Could you check a few things on this model? Use its own coordinates, in mm. Face numbers are marked on the shaded views. Coordinates: 2 decimals unless noted, no trailing zeros. Write each loop counter-clockwise with the first axis right and the second up, starting at its lowest first coordinate (ties: lowest second). Pieces come first, ordered by that corner, then holes. Notation, with made-up numbers: M 17.5,-31 L 69.5,-31 A11 cw 69.5,-15 Z; hole C 75,25.25 d10. An arc over 180 degrees is marked long. Write item = value, one per line.
Autodesk Inventor part; units mm, degrees
ref_plane "YZ Plane" through (0, 0, 0) normal (1, 0, 0) x (0, 1, 0)
ref_plane "XZ Plane" through (0, 0, 0) normal (0, 1, 0) x (-1, 0, 0)
ref_plane "XY Plane" through (0, 0, 0) normal (0, 0, 1) x (1, 0, 0)
sketch "Sketch1" plane through (0, 0, 0) normal (0, 1, 0) x (-1, 0, 0)
  line L0 (15, 7.5) -> (-15, 7.5)
  line L1 (-15, 7.5) -> (-15, -7.5)
  line L2 (-15, -7.5) -> (15, -7.5)
  line L3 (15, -7.5) -> (15, 7.5)
  line L4 (15, 7.5) -> (-15, -7.5) construction
  line L5 (-15, 7.5) -> (15, -7.5) construction
  line L6 (0, 7.5) -> (0, -7.5)
  line L7 (15, 0) -> (0, 0)
  circle A0 centre (7.5, 0) radius 2.25
  circle A1 centre (-7.7235, 0) radius 2
  dimension "d0" = 30
  dimension "d1" = 15
  dimension "d2" = 4.5
  dimension "d11" = 4
extrude "Extrusion1" add sketch "Sketch1" along normal blind 5 contours L3 L7 A0 L6 L0 | L6 L2 L1 L0 | L3 L2 L6 L7 A0
fillet "Fillet1" radius 3 4 edges at (-15, 2.5, 7.5) (-15, 2.5, -7.5) (15, 2.5, 7.5) (15, 2.5, -7.5)
properties part number "angulo"
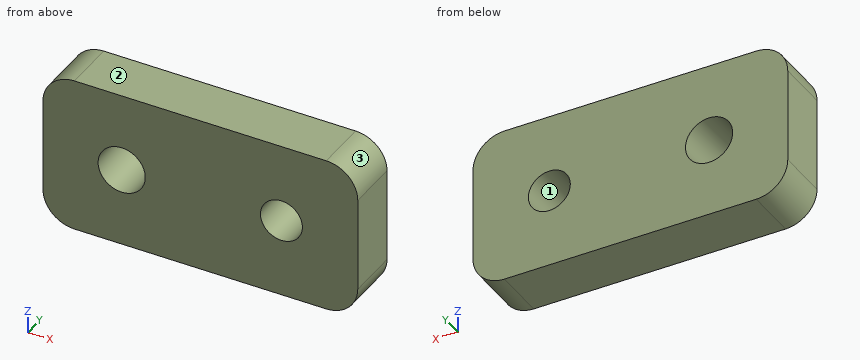
Item 1: Imagine slicing it at A-A (z = 0). Write out the boundary of the cut face in (x, y).
Numbers:
outline = M -15,0 L -9.75,0 L -9.75,5 L -15,5 Z; M -5.25,0 L 5.72,0 L 5.72,5 L -5.25,5 Z; M 9.72,0 L 15,0 L 15,5 L 9.72,5 Z
Item 2: If I drill on line 1 along Z through (x, y) = (-7.5, 2.1); line 2 along X through (y, z) = (3.9, -1.5); line 3 along Z through (x, y) = (-6.75, 2.7), over which ranges is the centre line in solid material (lowest first)?
Numbers:
line_1 = -7.5 to -2.25, 2.25 to 7.5
line_2 = -15 to -9.18, -5.82 to 6.4, 9.05 to 15
line_3 = -7.5 to -2.12, 2.12 to 7.5
Item 3: Imagine slicing it at D-D (x = 7). Write out the boundary of the cut face in (y, z).
Numbers:
outline = M 0,-7.5 L 5,-7.5 L 5,-1.86 L 0,-1.86 Z; M 0,1.86 L 5,1.86 L 5,7.5 L 0,7.5 Z
Item 4: I'm going to push a flat-ended pin straight in: P1, Ø1, axis at y = 4, z = 5.5, coming from the -X side. Where does the tip first touch, or does it pass through?
Numbers:
P1 = -14.96
Item 5: Imagine slicing it at B-B (x = -7.5). Write out the boundary of the cut face in (y, z), and give its area (3 significant figures).
Numbers:
outline = M 0,-7.5 L 5,-7.5 L 5,-2.25 L 0,-2.25 Z; M 0,2.25 L 5,2.25 L 5,7.5 L 0,7.5 Z
area = 52.5 mm²
Item 6: Imagine slicing it at C-C (y = 0.7). Write out the boundary of the cut face in (x, z).
Numbers:
outline = M -15,-4.5 A3 ccw -12,-7.5 L 12,-7.5 A3 ccw 15,-4.5 L 15,4.5 A3 ccw 12,7.5 L -12,7.5 A3 ccw -15,4.5 Z; hole C -7.5,0 d4.5; hole C 7.72,0 d4
Item 7: If we mould it in two halves opening along X, with no side actions, what happens to the marked faces 1, 2 and 3? For each: pulls with the +X half, pulls with the -X half, needs draft (parallel to the pull), parting line crosses it, or undercut.
Numbers:
face_1 = undercut
face_2 = needs draft
face_3 = pulls with the +X half
